Can you work these out from the model? Positions are in its coordinate system, mm. A direction names the side the tool comes from. Give positions to 0.01 mm unless a question says otherwise; leave off trailing zeros. Write each loop counter-clockwise with the first axis right and the second up, starting at its lowest first coordinate (ties: lowest second). Pieces come first, ordered by that corner, then holes. Notation, with made-up numbers: M 28.25,77.5 L 49.25,77.5 A13 cw 49.25,85.5 Z; hole C -30,0.5 d8. An arc over 180 degrees is marked long. Write each question's results on one line, items separated by ' | '.
Autodesk Inventor part; units mm, degrees
ref_plane "YZ Plane" through (0, 0, 0) normal (1, 0, 0) x (0, 1, 0)
ref_plane "XZ Plane" through (0, 0, 0) normal (0, 1, 0) x (-1, 0, 0)
ref_plane "XY Plane" through (0, 0, 0) normal (0, 0, 1) x (1, 0, 0)
sketch "Sketch1" plane through (0, 0, 0) normal (0, 0, 1) x (1, 0, 0)
  line L0 (-1.5875, 1.5875) -> (1.5875, 1.5875)
  line L1 (1.5875, 1.5875) -> (1.5875, -1.5875)
  line L2 (1.5875, -1.5875) -> (-1.5875, -1.5875)
  line L3 (-1.5875, -1.5875) -> (-1.5875, 1.5875)
  line L4 (-1.5875, 1.5875) -> (1.5875, -1.5875) construction
  line L5 (1.5875, 1.5875) -> (-1.5875, -1.5875) construction
  line L6 (-1.1875, -1.1875) -> (1.1875, -1.1875)
  line L7 (1.1875, -1.1875) -> (1.1875, 1.1875)
  line L8 (1.1875, 1.1875) -> (-1.1875, 1.1875)
  line L9 (-1.1875, 1.1875) -> (-1.1875, -1.1875)
  point P0 (0, 0)
  dimension "d0" = 3.175
  dimension "d1" = 0.4
extrude "Extrusion1" add sketch "Sketch1" along normal blind 100
properties part number "Rail" material "Aluminum 6061"
Item 1: I want a section at A-A, the plane x = -0.1. Please give me the cut outline in (y, z), and give its area (3 significant figures).
Geometry says:
outline: M -1.59,0 L -1.19,0 L -1.19,100 L -1.59,100 Z; M 1.19,0 L 1.59,0 L 1.59,100 L 1.19,100 Z | area: 80.0 mm2
Item 2: I'm going to push flat-ended pins straight in: pin 1 (1 mm diameter, centred on x = 0, y = 0.5, fed in from +Z); pin 2 (1 mm diameter, centred on x = 1, y = -1, fed in from +Z). Where does each tip first touch, or does it pass through?
Geometry says:
pin 1: passes through | pin 2: stops at z = 100
Item 3: If I drill on line 1 (Y direction, x = -1.05, z = 28.5), over which ranges is the centre line in solid material (lowest first)? Write a range as from..to.
Geometry says:
line 1: y = -1.59..-1.19, 1.19..1.59
Item 4: Thinking about a two-plate mould opening in X: for faces 1 (the face through (1.188, 0, 49)), 2 (the face through (0, -1.588, 49)), 3 (the face through (-1.588, 0, 49)), which applies, +X half, -X half, draft (parallel to the pull), parting line (faces both ways), or undercut?
Geometry says:
face 1: undercut | face 2: draft | face 3: -X half
Item 5: I want a section at C-C, the plane z = 76. Please give me the cut outline in (x, y), and give its area (3 significant figures).
Geometry says:
outline: M -1.59,-1.59 L 1.59,-1.59 L 1.59,1.59 L -1.59,1.59 Z; hole M -1.19,-1.19 L 1.19,-1.19 L 1.19,1.19 L -1.19,1.19 Z | area: 4.44 mm2
Item 6: For faces 4 (the face through (1.4, 0, 0)), 5 (the face through (0, -1.188, 49)), which set-ups out of +Z, -Z, +X, -X, +Y, -Y let a thin tool reach every point of the face, with its end or its side?
Geometry says:
face 4: -Z, +X, -X, +Y, -Y | face 5: +Z, -Z
